Geometry check sheet. Reference: the model listing, model coordinates, mm. A direction names the side the tool comes from. Round coordinates to 2 decimals unless told otherwise and drop trailing zeros. Write each loop counter-clockwise with the first axis right and the second up, starting at its lowest first coordinate (ties: lowest second). Pieces come first, ordered by that corner, then holes. Notation, with made-up numbers: (37, 10) -> (83, 10) arc R22 cw to (83, 47) -> close; hole circle Ø7 at (81.5, 21). An arc over 180 degrees is marked (long way). One line per question, with ' | ' between items.
```python
from build123d import *

# Parameters (mm, degrees)
SKETCH1_R           = 8
BOSS_EXTRUDE1_DEPTH = 115
SKETCH2_R           = 10
BOSS_EXTRUDE2_DEPTH = 10
BOSS_EXTRUDE3_START = 10
SKETCH3_R           = 10
BOSS_EXTRUDE3_DEPTH = 10
SKETCH4_R           = 8
BOSS_EXTRUDE4_DEPTH = 16
SKETCH5_R           = 7.5
BOSS_EXTRUDE5_DEPTH = 16
SKETCH6_R           = 3
CUT_EXTRUDE1_DEPTH  = 75
SKETCH7_R           = 4.5
CUT_EXTRUDE2_DEPTH  = 4
CUT_EXTRUDE3_START  = -16
CUT_EXTRUDE3_DEPTH  = 16
SKETCH9_R           = 3
CUT_EXTRUDE4_DEPTH  = 143.256810049


with BuildPart() as part:
    # Sketch1 → Boss-Extrude1 (new body)
    with BuildSketch(Plane.XY):
        Circle(SKETCH1_R)
    extrude(amount=BOSS_EXTRUDE1_DEPTH)

    # Sketch2 → Boss-Extrude2 (add)
    with BuildSketch(Plane(origin=(0, 0, 0), x_dir=(-1, 0, 0), z_dir=(0, 0, -1))):
        Circle(SKETCH2_R)
    extrude(amount=BOSS_EXTRUDE2_DEPTH)

    # Sketch3 → Boss-Extrude3 (add)
    with BuildSketch(Plane.XY.offset(115).offset(BOSS_EXTRUDE3_START)):
        with Locations(Location((0, 0, 0), (0, 0, 180))):
            Circle(SKETCH3_R)
    extrude(amount=-BOSS_EXTRUDE3_DEPTH)

    # Sketch4 → Boss-Extrude4 (add)
    with BuildSketch(Plane.XY.offset(125)):
        with Locations(Location((0, 0, 0), (0, 0, 180))):
            Circle(SKETCH4_R)
    extrude(amount=BOSS_EXTRUDE4_DEPTH)

    # Sketch5 → Boss-Extrude5 (add)
    with BuildSketch(Plane(origin=(0, 0, -10), x_dir=(-1, 0, 0), z_dir=(0, 0, -1))):
        Circle(SKETCH5_R)
    extrude(amount=BOSS_EXTRUDE5_DEPTH)

    # Sketch6 → Cut-Extrude1 (cut)
    with BuildSketch(Plane.XY.offset(141)):
        Circle(SKETCH6_R)
    extrude(amount=-CUT_EXTRUDE1_DEPTH, mode=Mode.SUBTRACT)

    # Sketch7 → Cut-Extrude2 (cut)
    with BuildSketch(Plane(origin=(0, 10, 0), x_dir=(-1, 0, 0), z_dir=(0, 1, 0))):
        with Locations(Location((0, 120, 0), (0, 0, 90))):
            Circle(SKETCH7_R)
        with Locations(Location((0, -5, 0), (0, 0, 90))):
            Circle(SKETCH7_R)
    extrude(amount=-CUT_EXTRUDE2_DEPTH, mode=Mode.SUBTRACT)

    # Sketch8 → Cut-Extrude3 (cut)
    with BuildSketch(Plane(origin=(0, 0, -26), x_dir=(-1, 0, 0), z_dir=(0, 0, -1)).offset(CUT_EXTRUDE3_START)):
        with BuildLine():
            Line((-6, 4.5), (-6, -4.5))
            ThreePointArc((-6, -4.5), (-7.5, 0), (-6, 4.5))
        make_face()
        with BuildLine():
            Line((6, 4.5), (6, -4.5))
            ThreePointArc((6, -4.5), (7.5, 0), (6, 4.5))
        make_face()
    extrude(amount=CUT_EXTRUDE3_DEPTH, mode=Mode.SUBTRACT)

    # Sketch9 → Cut-Extrude4 (cut, through all)
    with BuildSketch(Plane(origin=(6, 0, 0), x_dir=(0, 0, -1), z_dir=(1, 0, 0))):
        with Locations((19, 0)):
            Circle(SKETCH9_R)
    extrude(amount=-CUT_EXTRUDE4_DEPTH, mode=Mode.SUBTRACT)


solid = part.part
```
(1) Go/stop test with flat-tipped pins: pin 1 (4.5 mm diameter, centred on x = 1.5, z = 118, fed in from +Y); pin 2 (4 mm diameter, centred on y = 7, z = 35, fed in from +X) (3 decimals); pin 3 (8 mm diameter, centred on y = 3, z = 6, fed in from -X). Record where each tip stops, or that it passes through.
Resolved:
pin 1: stops at y = 9.89 | pin 2: stops at x = 6.245 | pin 3: stops at x = -8
(2) Sectioned sample at D-D on z = 63. Record the cut outline in (x, y).
Resolved:
outline: circle Ø16 at (0, 0)
(3) Sectioned sample at C-C on z = 120. Record the cut outline in (x, y).
Resolved:
outline: (-4.5, 6) -> (-4.5, 8.93) arc R10 ccw (long way) to (4.5, 8.93) -> (4.5, 6) -> close; hole circle Ø6 at (0, 0)
(4) Access from +Z, -Z, +X, -X, +Y, -Y to the whole of each face (thin tool, end or side, straight path). Record for faces 1 (the flat face through (-6, 1, -16)), 2 (the cylindrical face through (1.352, 7.584, -0.708)), 3 (the cylindrical face through (-3, 0, 104)).
Resolved:
face 1: -Z, -X, +Y, -Y | face 2: +Y | face 3: +Z
(5) Material ranges on line 1 (Z direction, x = -7.5, y = 3.5); line 2 (X direction, y = 8, z = -5); line 3 (Y direction, x = 0, z = 121), recorded low to high.
Resolved:
line 1: z = -10 to 0, 115 to 125 | line 2: x = -6 to -4.5, 4.5 to 6 | line 3: y = -10 to -3, 3 to 6
(6) Sectioned sample at A-A on y = 0. Record the cut outline in (x, z).
Resolved:
outline: (-10, -10) -> (-6, -10) -> (-6, -16) -> (6, -16) -> (6, -10) -> (10, -10) -> (10, 0) -> (8, 0) -> (8, 115) -> (10, 115) -> (10, 125) -> (8, 125) -> (8, 141) -> (3, 141) -> (3, 66) -> (-3, 66) -> (-3, 141) -> (-8, 141) -> (-8, 125) -> (-10, 125) -> (-10, 115) -> (-8, 115) -> (-8, 0) -> (-10, 0) -> close; (-6, -26) -> (6, -26) -> (6, -22) -> (-6, -22) -> close
(7) Draft check along Z on faces 4 (the flat face through (0, 8.2, 0)), 5 (the cylindrical face through (1.73, 7.81, 132.89)), 6 (the flat face through (0, 0, 66)). Enter one of: +Z half, -Z half, draft (parallel to the pull), parting line (faces both ways), or undercut.
Resolved:
face 4: undercut | face 5: draft | face 6: +Z half
